Autodesk Inventor part; units mm, degrees
ref_plane "YZ Plane" through (0, 0, 0) normal (1, 0, 0) x (0, 1, 0)
ref_plane "XZ Plane" through (0, 0, 0) normal (0, 1, 0) x (-1, 0, 0)
ref_plane "XY Plane" through (0, 0, 0) normal (0, 0, 1) x (1, 0, 0)
sketch "Sketch1" plane through (0, 0, 0) normal (1, 0, 0) x (0, 1, 0)
  line L0 (13.6162, 14.8297) -> (-11.3125, 14.8297)
  line L1 (-11.3125, 14.8297) -> (-11.3125, -13.9659)
  line L2 (-11.3125, -13.9659) -> (13.6162, -13.9659)
  line L3 (13.6162, -13.9659) -> (13.6162, 14.8297)
extrude "Extrusion1" add sketch "Sketch1" along normal mid plane 25.4
sketch "Sketch2" plane through (12.7, 0, 0) normal (1, 0, 0) x (0, 0, -1)
  line L0 (-12.1558, 10.6955) -> (11.4154, 10.6955)
  line L1 (11.4154, 10.6955) -> (11.4154, -9.0912)
  line L2 (11.4154, -9.0912) -> (-12.1558, -9.0912)
  line L3 (-12.1558, -9.0912) -> (-12.1558, 10.6955)
  point P0 (0, 0)
extrude "Extrusion2" cut sketch "Sketch2" against normal blind 25.4
sketch "Sketch3" plane through (12.7, 0, 0) normal (1, 0, 0) x (0, 0, -1)
  line L0 (-14.8297, -11.3125) -> (13.9659, -11.3125)
  line L1 (-8.621, -11.3125) -> (8.8651, -11.3125)
  line L2 (8.8651, -11.3125) -> (8.8651, -32.2195)
  line L3 (8.8651, -32.2195) -> (-8.621, -32.2195)
  line L4 (-8.621, -32.2195) -> (-8.621, -11.3125)
  point P0 (0, 0)
extrude "Extrusion3" add sketch "Sketch3" against normal blind 25.4
sketch "Sketch4" plane through (12.7, 0, 0) normal (1, 0, 0) x (0, 0, -1)
  line L0 (-6.8955, -13.2073) -> (6.5094, -13.2073)
  line L1 (6.5094, -13.2073) -> (6.5094, -30.471)
  line L2 (6.5094, -30.471) -> (-6.8955, -30.471)
  line L3 (-6.8955, -30.471) -> (-6.8955, -13.2073)
  point P0 (0, 0)
extrude "Extrusion4" cut sketch "Sketch4" against normal blind 25.4
sketch "Sketch6" plane through (12.7, -32.2195, -8.8651) normal (0, -1, 0) x (1, 0, 0)
  point P0 (-12.7, 8.8651)
Design review of the part built by this model. Coordinates are the model's own, in mm. A direction names the side the tool comes from. Give positions to 0.01 mm unless a question says otherwise; leave off trailing zeros. Write each loop counter-clockwise with the first axis right and the second up, starting at its lowest first coordinate (ties: lowest second). Pieces come first, ordered by that corner, then holes. Notation, with made-up numbers: M -29,24.25 L 9,24.25 A28 ccw 9,56.25 Z; hole C -38.75,42 d1. An arc over 180 degrees is marked long. Answer as a JSON object with one key per item and string values. Group by question number.
1) We need section C-C (x = -0.75). Give the boundary of the cut face in (y, z), and give its area (3 significant figures).
2) For line 1 along Y through (x, z) = (7, -5.75); line 2 along Z through (x, y) = (1, -7.5); line 3 along Z through (x, y) = (1.25, -17), list the stretches that pass through material, from the lowest coordinate up.
3) Mouldability with a two-part tool opening along Z and no side actions: class faces 6 (the face through (0, -22, 8.621)), 7 (the face through (0, -22, 6.896)), 8 (the face through (0, -32.219, 0)) as released by +Z, released by -Z, zero draft, split by the parting line, or undercut.
4) Clearance check with flat-ended pins moving along their axes: pin 1 Ø10 at (y, z) = (-6, 6) entering from +X; pin 2 Ø2.5 at (x, z) = (1, -12.5) entering from -Y; pin 3 Ø8 at (y, z) = (-3, -0.5) entering from +X; pin 4 Ø10.5 at (x, y) = (-4.5, -21.5) entering from -Z. State where each tip first meets the part, or that it passes through.
5) We need section A-A (y = -27). Give the boundary of the cut face in (x, z).
6) Tool access review of faces 1 (the face through (-12.7, -9.4, 1.6)), 2 (the face through (0, -11.312, 12)), 3 (the face through (0, 13.616, 0)), 4 (the face through (0, 1, 12.156)), 5 (the face through (0, -22, -8.865)): name each direction out of +Z, -Z, +X, -X, +Y, -Y from which nothing blocks a thin tool from reaching the whole face with its end or side.
7) We need section B-B (z = -10.5). Give the boundary of the cut face in (x, y), and give its area (3 significant figures).
8) We need section D-D (z = -1.25). Give the boundary of the cut face in (x, y).
Answer key:
{
 "1": {"outline": "M -32.22,-8.87 L -11.31,-8.87 L -11.31,-13.97 L 13.62,-13.97 L 13.62,14.83 L -11.31,14.83 L -11.31,8.62 L -32.22,8.62 Z; hole M -30.47,-6.51 L -13.21,-6.51 L -13.21,6.9 L -30.47,6.9 Z; hole M -9.09,-11.42 L 10.7,-11.42 L 10.7,12.16 L -9.09,12.16 Z", "area": "386 mm²"},
 "2": {"line 1": "y = -32.22 to -30.47, -13.21 to -9.09, 10.7 to 13.62", "line 2": "z = -13.97 to -11.42, 12.16 to 14.83", "line 3": "z = -8.87 to -6.51, 6.9 to 8.62"},
 "3": {"face 6": "released by +Z", "face 7": "undercut", "face 8": "zero draft"},
 "4": {"pin 1": "stops at x = 12.7", "pin 2": "stops at y = -11.31", "pin 3": "passes through", "pin 4": "stops at z = -8.87"},
 "5": {"outline": "M -12.7,-8.87 L 12.7,-8.87 L 12.7,-6.51 L -12.7,-6.51 Z; M -12.7,6.9 L 12.7,6.9 L 12.7,8.62 L -12.7,8.62 Z"},
 "6": {"face 1": "+Z, -Z, -X, +Y, -Y", "face 2": "+Z, +X, -X, -Y", "face 3": "+Z, -Z, +X, -X, +Y", "face 4": "+X, -X", "face 5": "-Z, +X, -X, -Y"},
 "7": {"outline": "M -12.7,-11.31 L 12.7,-11.31 L 12.7,-9.09 L -12.7,-9.09 Z; M -12.7,10.7 L 12.7,10.7 L 12.7,13.62 L -12.7,13.62 Z", "area": "131 mm²"},
 "8": {"outline": "M -12.7,-32.22 L 12.7,-32.22 L 12.7,-30.47 L -12.7,-30.47 Z; M -12.7,-13.21 L 12.7,-13.21 L 12.7,-9.09 L -12.7,-9.09 Z; M -12.7,10.7 L 12.7,10.7 L 12.7,13.62 L -12.7,13.62 Z"}
}
